Source: three-view drawing plus pictorial views. Frame: mm from the lowest corner of the part. A direction names the side the tool comes from. Round coordinates to 2 decimals unless told otherwise and drop trailing zeros. Write each loop counter-clockwise with the first axis right and the second up, starting at its lowest first coordinate (ties: lowest second). Pieces come first, ordered by that corner, then holes.
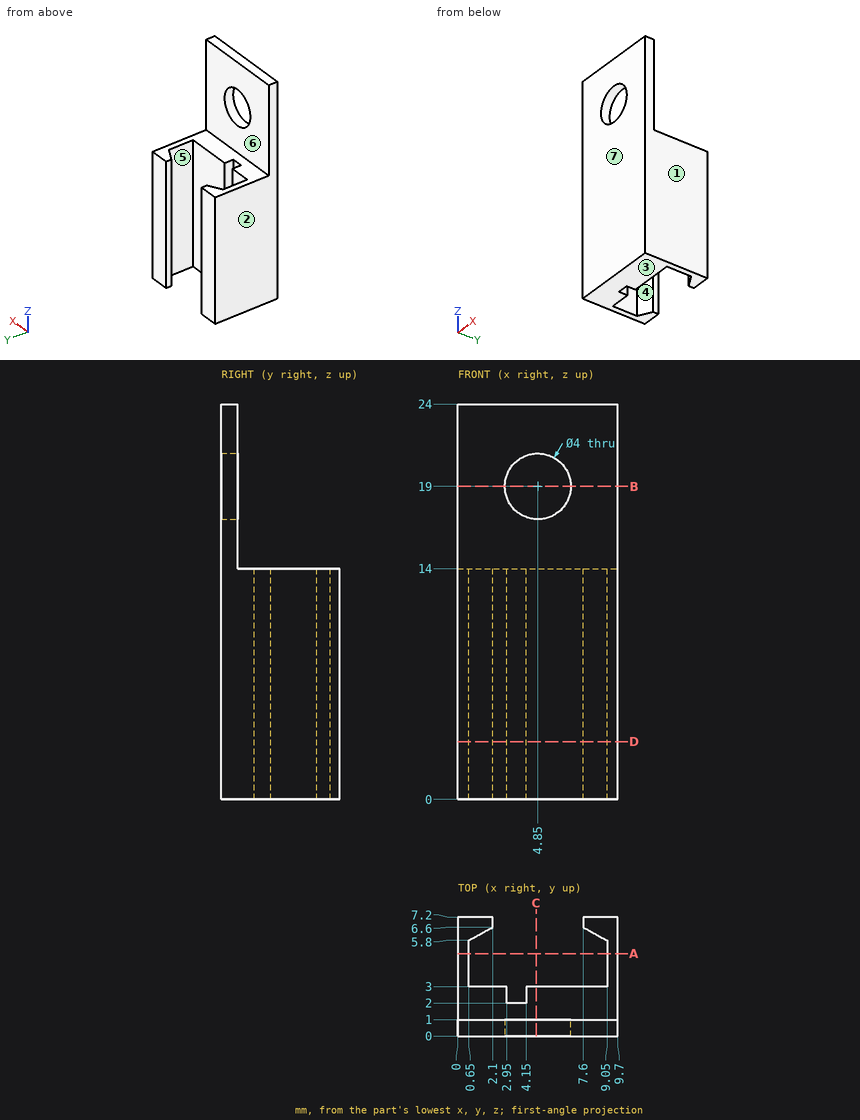
1) Line query: probe 1 along X at (y, z) = (4.25, 11.25); probe 2 along Z at (x, y) = (4.85, 0.35); probe 3 along X at (y, z) = (2.25, 13). Output: solid intervals per line, ascending.
2) Section C-C on x = 4.75. Output: boundary loops of the cut face in (y, z).
3) Reachability of the marked faces 5, 6 and 7 from +Z, -Z, +X, -X, +Y, -Y: full face, straight path, thin tool, end or side. Return the list, or none.
4) Section B-B on z = 19. Output: boundary loops of the cut face in (x, y).
5) Draft query along X for the marked faces 1, 2, 3 and 4. Return one class per face: pulls with the +X half, pulls with the -X half, needs draft (parallel to the pull), parting line crosses it, or undercut.
6) Section A-A on y = 5. Output: boundary loops of the cut face in (x, z), plus the area to 3 significant figures.
7) First-contact query: P1, Ø1.5, axis at x = 6.5, z = 7.5, coming from the +Y side. Flat tip, straight axial feed; report the tip coordinate or a pass-through.
8) Section D-D on z = 3.5. Output: boundary loops of the cut face in (x, y), plus the area to 3 significant figures.
Filled in:
1. probe 1: x = 0 to 0.65, 9.05 to 9.7
1. probe 2: z = 0 to 17, 21 to 24
1. probe 3: x = 0 to 2.95, 4.15 to 9.7
2. outline: (0, 0) - (3, 0) - (3, 14) - (1, 14) - (1, 17) - (0, 17) - close; (0, 21) - (1, 21) - (1, 24) - (0, 24) - close
3. face 5: +Z, -Z
3. face 6: +Z, +X, -X, +Y
3. face 7: +Z, -Z, +X, -X, -Y
4. outline: (0, 0) - (2.85, 0) - (2.85, 1) - (0, 1) - close; (6.85, 0) - (9.7, 0) - (9.7, 1) - (6.85, 1) - close
5. face 1: pulls with the +X half
5. face 2: pulls with the -X half
5. face 3: needs draft
5. face 4: undercut
6. outline: (0, 0) - (0.65, 0) - (0.65, 14) - (0, 14) - close; (9.05, 0) - (9.7, 0) - (9.7, 14) - (9.05, 14) - close
6. area: 18.2 mm2
7. P1: stops at y = 3
8. outline: (0, 0) - (9.7, 0) - (9.7, 7.2) - (7.6, 7.2) - (7.6, 6.6) - (9.05, 5.8) - (9.05, 3) - (4.15, 3) - (4.15, 2) - (2.95, 2) - (2.95, 3) - (0.65, 3) - (0.65, 5.8) - (2.1, 6.6) - (2.1, 7.2) - (0, 7.2) - close
8. area: 36.3 mm2
